For this review, take the finished solid that the model builds, in its own axes (mm). Coordinates: 2 decimals unless noted, no trailing zeros. Loops run counter-clockwise (first coordinate to the right, second up) from the corner with the lowest first, then second, coordinate; pieces in that order, holes last. Notation, with made-up numbers: (-19, 88) -> (28, 88) arc R32 cw to (28, 125) -> close; hole circle Ø4 at (-29, -32.5). An arc over 180 degrees is marked (long way). Use a Markdown table: item, result.
from build123d import *

# Parameters (mm, degrees)
F0_W     = 50
F0_H     = 30
F0_W_2   = 22
F0_H_2   = 26
F1_DEPTH = 680


with BuildPart() as f1:
    # F0 (on Right) → F1 (new body)
    with BuildSketch(Plane.YZ):
        Rectangle(F0_W, F0_H)
        with Locations((-12, 0)):
            Rectangle(F0_W_2, F0_H_2, mode=Mode.SUBTRACT)
        with Locations((12, 0)):
            Rectangle(F0_W_2, F0_H_2, mode=Mode.SUBTRACT)
    extrude(amount=F1_DEPTH)


solid = f1.part
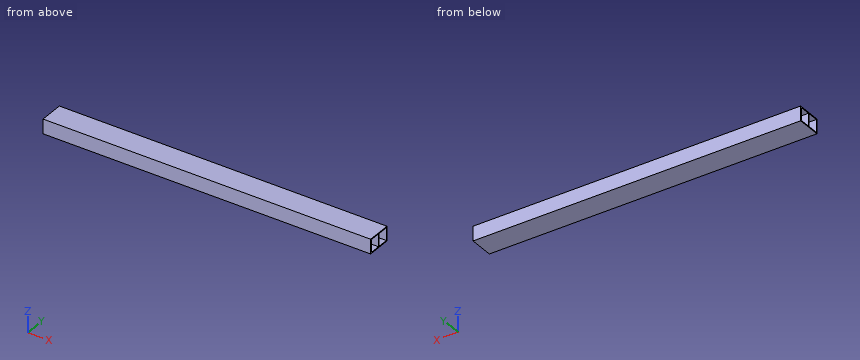
(1) Take a section at C-C on z = -6.5. Write out the cut boundary in (x, y).
Found:
| item | result |
|---|---|
| outline | (0, -25) -> (680, -25) -> (680, -23) -> (0, -23) -> close; (0, -1) -> (680, -1) -> (680, 1) -> (0, 1) -> close; (0, 23) -> (680, 23) -> (680, 25) -> (0, 25) -> close |
(2) Take a section at A-A on y = -16.5. Write out the cut boundary in (x, z), plus the area to 3 significant figures.
Found:
| item | result |
|---|---|
| outline | (0, -15) -> (680, -15) -> (680, -13) -> (0, -13) -> close; (0, 13) -> (680, 13) -> (680, 15) -> (0, 15) -> close |
| area | 2,720 mm^2 |
(3) Take a section at B-B on x = 139. Write out the cut boundary in (y, z), plus the area to 3 significant figures.
Found:
| item | result |
|---|---|
| outline | (-25, -15) -> (25, -15) -> (25, 15) -> (-25, 15) -> close; hole (-23, -13) -> (-1, -13) -> (-1, 13) -> (-23, 13) -> close; hole (1, -13) -> (23, -13) -> (23, 13) -> (1, 13) -> close |
| area | 356 mm^2 |
(4) For pin 1 Ø1 at (y, z) = (5, 12) entering from +X, flat-tipped, find the tip position at first contact; note if it passes through.
Found:
| item | result |
|---|---|
| pin 1 | passes through |
(5) For line 1 along Y through (x, z) = (583, 0.75); line 2 along Z through (x, y) = (240, 2), list the stretches that pass through material, from the lowest coordinate up.
Found:
| item | result |
|---|---|
| line 1 | y = -25 to -23, -1 to 1, 23 to 25 |
| line 2 | z = -15 to -13, 13 to 15 |
